Could you check a few things on this model? Use its own coordinates, in mm. Coordinates: 2 decimals unless noted, no trailing zeros. Loops run counter-clockwise (first coordinate to the right, second up) from the corner with the lowest first, then second, coordinate; pieces in that order, holes last. Notation, with made-up numbers: (89.5, 69.25) -> (111.5, 69.25) arc R10 ccw to (111.5, 76.25) -> close; hole circle Ø1 at (-21, 60.25). An arc over 180 degrees is marked (long way). One line per question, with ' | ' between items.
```python
from build123d import *

# Parameters (mm, degrees)
F0_R     = 11
F1_DEPTH = 4.5
F4_SIZE  = 2
F5_SIZE  = 1


# Not quite as in the source:
# - a feature of the source that left no trace in its solid (it failed there, or was rolled back) is left out


with BuildPart() as f1:
    # F0 (on Top) → F1 (new body, symmetric)
    with BuildSketch(Plane.XY):
        with BuildLine():
            ThreePointArc((-24.248711306, 3), (-38.9711431703, -22.5), (-9.5262794416, -22.5))
            ThreePointArc((-9.5262794416, -22.5), (0, -17), (9.5262794416, -22.5))
            ThreePointArc((9.5262794416, -22.5), (38.9711431703, -22.5), (24.248711306, 3))
            ThreePointArc((24.248711306, 3), (14.7224318643, 8.5), (14.7224318643, 19.5))
            ThreePointArc((14.7224318643, 19.5), (0, 45), (-14.7224318643, 19.5))
            ThreePointArc((-14.7224318643, 19.5), (-14.7224318643, 8.5), (-24.248711306, 3))
        make_face()
        with Locations((-24.248711306, -14)):
            Circle(F0_R, mode=Mode.SUBTRACT)
        with Locations((24.248711306, -14)):
            Circle(F0_R, mode=Mode.SUBTRACT)
        Circle(F0_R, mode=Mode.SUBTRACT)
        with Locations((0, 28)):
            Circle(F0_R, mode=Mode.SUBTRACT)
    extrude(amount=F1_DEPTH, both=True)

    # F4
    f4_edges = [f1.edges().sort_by_distance(p)[0] for p in [
        (-38.971143, -22.5, 4.5),
        (-38.971143, -22.5, -4.5),
        (-14.722432, 8.5, -4.5),
        (-14.722432, 8.5, 4.5),
        (0, 45, -4.5),
        (0, 45, 4.5),
        (14.722432, 8.5, -4.5),
        (14.722432, 8.5, 4.5),
        (38.971143, -22.5, -4.5),
        (38.971143, -22.5, 4.5),
        (0, -17, -4.5),
        (0, -17, 4.5),
    ]]
    chamfer(f4_edges, length=F4_SIZE)

    # F5
    f5_edges = [f1.edges().sort_by_distance(p)[0] for p in [
        (-35.248711, -14, 4.5),
        (-13.248711, -14, 0),
        (-35.248711, -14, -4.5),
        (-11, 0, 4.5),
        (11, 0, 0),
        (-11, 0, -4.5),
        (-11, 28, 4.5),
        (11, 28, 0),
        (-11, 28, -4.5),
        (13.248711, -14, 4.5),
        (35.248711, -14, 0),
        (13.248711, -14, -4.5),
    ]]
    chamfer(f5_edges, length=F5_SIZE)


solid = f1.part
```
Q1. Imagine slicing it at B-B on x = 0. Write out the boundary of the cut face in (y, z), plus the area to 3 significant figures.
Values follow:
outline: (-17, -2.5) -> (-15, -4.5) -> (-12, -4.5) -> (-11, -3.5) -> (-11, 3.5) -> (-12, 4.5) -> (-15, 4.5) -> (-17, 2.5) -> close; (11, -3.5) -> (12, -4.5) -> (16, -4.5) -> (17, -3.5) -> (17, 3.5) -> (16, 4.5) -> (12, 4.5) -> (11, 3.5) -> close; (39, -3.5) -> (40, -4.5) -> (43, -4.5) -> (45, -2.5) -> (45, 2.5) -> (43, 4.5) -> (40, 4.5) -> (39, 3.5) -> close | area: 150 mm2
Q2. We'd pull the mould along Y, two halves only. Please class faces 1 (the face through (0, 45, 0)), 2 (the face through (0, -17, 0)), 3 (the face through (0, 13, 4.5)): released by +Y, released by -Y, zero draft, split by the parting line, or undercut.
Values follow:
face 1: undercut | face 2: released by -Y | face 3: zero draft
Q3. Imagine slicing it at C-C on y = 28. Write out the boundary of the cut face in (x, z).
Values follow:
outline: (-17, -2.5) -> (-15, -4.5) -> (-12, -4.5) -> (-11, -3.5) -> (-11, 3.5) -> (-12, 4.5) -> (-15, 4.5) -> (-17, 2.5) -> close; (11, -3.5) -> (12, -4.5) -> (15, -4.5) -> (17, -2.5) -> (17, 2.5) -> (15, 4.5) -> (12, 4.5) -> (11, 3.5) -> close
Q4. Imagine slicing it at D-D on z = 0.5. Write out the boundary of the cut face in (x, y), plus the area to 3 significant figures.
Values follow:
outline: (-24.25, 3) arc R17 ccw (long way) to (-9.53, -22.5) arc R11 cw to (9.53, -22.5) arc R17 ccw (long way) to (24.25, 3) arc R11 cw to (14.72, 19.5) arc R17 ccw (long way) to (-14.72, 19.5) arc R11 cw to start; hole circle Ø22 at (-24.25, -14); hole circle Ø22 at (0, 0); hole circle Ø22 at (0, 28); hole circle Ø22 at (24.25, -14) | area: 1,950 mm2
Q5. For pin 1 (2 mm diameter, centred on y = -12.5, z = 3, fed in from +X); pin 2 (2 mm diameter, centred on x = 20, z = 3, fed in from +Y); pin 3 (1.5 mm diameter, centred on x = 10.5, y = -0.5, fed in from -Z); pin 4 (10 mm diameter, centred on x = -26.5, y = -22.5, fed in from +Z), each with a flat end and sliding along its axis, tell me the tip position at first contact or that it passes through.
Values follow:
pin 1: stops at x = 41.24 | pin 2: stops at y = 4.26 | pin 3: stops at z = -3.76 | pin 4: stops at z = 4.5
Q6. Please list where these lines run through material, in increasing order: L1, parallel to Y at x = -0.5, z = 1; L2, parallel to Y at x = -1, z = 3; L3, parallel to X at y = 28.5, z = -1. Write a range as [from, to].
Values follow:
L1: y = [-17.01, -10.99], [10.99, 17.01], [38.99, 44.99] | L2: y = [-16.54, -10.95], [10.95, 17.05], [38.95, 44.47] | L3: x = [-16.99, -10.99], [10.99, 16.99]
Q7. Imagine slicing it at A-A on y = -14. Write out the boundary of the cut face in (x, z).
Values follow:
outline: (-41.25, -2.5) -> (-39.25, -4.5) -> (-36.25, -4.5) -> (-35.25, -3.5) -> (-35.25, 3.5) -> (-36.25, 4.5) -> (-39.25, 4.5) -> (-41.25, 2.5) -> close; (-13.25, -3.5) -> (-12.25, -4.5) -> (12.25, -4.5) -> (13.25, -3.5) -> (13.25, 3.5) -> (12.25, 4.5) -> (-12.25, 4.5) -> (-13.25, 3.5) -> close; (35.25, -3.5) -> (36.25, -4.5) -> (39.25, -4.5) -> (41.25, -2.5) -> (41.25, 2.5) -> (39.25, 4.5) -> (36.25, 4.5) -> (35.25, 3.5) -> close
